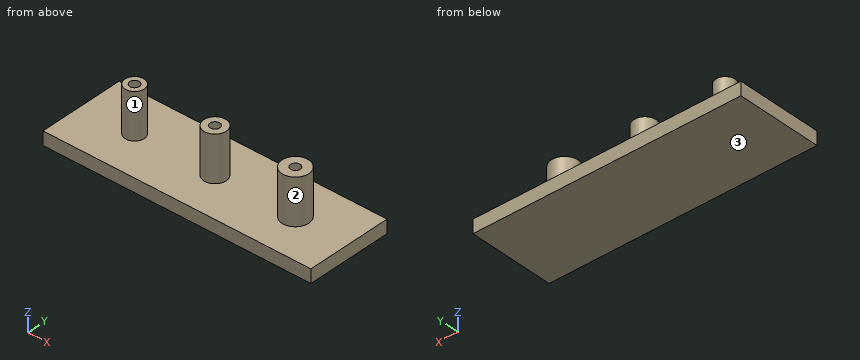
Autodesk Fusion 360 part; units mm, degrees
sketch "Esquisse1" plane through (0, 0, 0) normal (0, 0, 1) x (1, 0, 0)
  line L0 (0, 0) -> (50, 0)
  line L1 (50, 0) -> (50, 16)
  line L2 (50, 16) -> (0, 16)
  line L3 (0, 16) -> (0, 0)
  dimension "d7" = 50
  dimension "d8" = 16
extrude "Extrusion1" add sketch "Esquisse1" along normal blind 2.5
sketch "Esquisse2" plane through (0, 0, 2.5) normal (0, 0, 1) x (-1, 0, 0)
  line L0 (0, -16) -> (0, 0)
  line L1 (0, 0) -> (-50, 0)
  line L2 (-50, 0) -> (-50, -16)
  line L3 (-50, -16) -> (0, -16)
  circle A0 centre (-10, -8) radius 1.8
  dimension "d11" = 3.6
  dimension "d12" = 8
  dimension "d13" = 10
extrude "Extrusion2" add sketch "Esquisse2" along normal blind 8.5 contours A0
sketch "Esquisse3" plane through (0, 0, 2.5) normal (0, 0, 1) x (-1, 0, 0)
  circle A0 centre (-10, -8) radius 1.8
  line L0 (0, -16) -> (0, 0)
  line L1 (0, 0) -> (-50, 0)
  line L2 (-50, 0) -> (-50, -16)
  line L3 (-50, -16) -> (0, -16)
  circle A1 centre (-25, -8) radius 2.1
  dimension "d16" = 4.2
  dimension "d17" = 8
  dimension "d18" = 25
extrude "Extrusion3" add sketch "Esquisse3" along normal blind 8.5 contours A1
sketch "Esquisse4" plane through (0, 0, 2.5) normal (0, 0, 1) x (-1, 0, 0)
  circle A0 centre (-25, -8) radius 2.1
  circle A1 centre (-10, -8) radius 1.8
  line L0 (0, -16) -> (0, 0)
  line L1 (0, 0) -> (-50, 0)
  line L2 (-50, 0) -> (-50, -16)
  line L3 (-50, -16) -> (0, -16)
  circle A2 centre (-40, -8) radius 2.5
  dimension "d21" = 5
  dimension "d22" = 8
  dimension "d23" = 40
extrude "Extrusion4" add sketch "Esquisse4" along normal blind 8.5 contours A2
sketch "Esquisse5" plane through (0, 0, 11) normal (0, 0, 1) x (-1, 0, 0)
  circle A0 centre (-10, -8) radius 1.8
  circle A1 centre (-10, -8) radius 0.9
  dimension "d26" = 1.8
extrude "Extrusion5" cut sketch "Esquisse5" against normal blind 6 contours A1
pattern_linear "Réseau R1" count 3 spacing 15 along (1, 0, 0) of "Extrusion5"
equation "l_plaque = 50 mm"
equation "w_plaque = 16 mm"
equation "ep_plaque = 2.5 mm"
equation "h_plot = 8.5 mm"
equation "d_pilote = 1.8 mm"
equation "p_pilote = 6 mm"
equation "d7 = l_plaque"
equation "d8 = w_plaque"
equation "d9 = ep_plaque"
equation "d14 = h_plot"
equation "d19 = h_plot"
equation "d24 = h_plot"
equation "d26 = d_pilote"
Source: CAD feature listing. Evaluate the final solid. Frame: model axes, mm. Face numbers are marked on the shaded views. Coordinates: 2 decimals unless noted, no trailing zeros. Order: outer loops, then holes, each group sorted by start corner. A loop starts at its lowest first (then second) coordinate and runs counter-clockwise, first axis right, second up. Notation, with made-up numbers: (75, -25.5) - (94, -25.5) arc R26 ccw to (94, -4.5) - close; hole circle Ø1 at (10.25, -22.75). An arc over 180 degrees is marked (long way). One line per item, written item: value.
1) Contact query for flat-ended pins moving along their axis: pin 1 (1.6 mm diameter, centred on x = 40, y = 8, fed in from +Z); pin 2 (3 mm diameter, centred on x = 20.5, y = 10.5, fed in from +Z); pin 3 (2 mm diameter, centred on y = 10.5, z = 9.5, fed in from +X). Output: stop coordinate, or through.
Computed values:
pin 1: stops at z = 5
pin 2: stops at z = 2.5
pin 3: stops at x = 42
2) Cut plane A-A on z = 7. Output: boundary loops of the cut face in (x, y), plus the area to 3 significant figures.
Computed values:
outline: circle Ø3.6 at (10, 8); circle Ø4.2 at (25, 8); circle Ø5 at (40, 8); hole circle Ø1.8 at (10, 8); hole circle Ø1.8 at (25, 8); hole circle Ø1.8 at (40, 8)
area: 36.0 mm^2
3) Ray query, line 1 (X direction, y = 8, z = 6.75); line 2 (Y direction, x = 40, z = 9); line 3 (Y direction, x = 25, z = 9.25). Return the intervals inside material, ascending. Write a range as [from, to].
Computed values:
line 1: x = [8.2, 9.1], [10.9, 11.8], [22.9, 24.1], [25.9, 27.1], [37.5, 39.1], [40.9, 42.5]
line 2: y = [5.5, 7.1], [8.9, 10.5]
line 3: y = [5.9, 7.1], [8.9, 10.1]
4) Cut plane C-C on x = 25. Output: boundary loops of the cut face in (y, z), plus the area to 3 significant figures.
Computed values:
outline: (0, 0) - (16, 0) - (16, 2.5) - (10.1, 2.5) - (10.1, 11) - (8.9, 11) - (8.9, 5) - (7.1, 5) - (7.1, 11) - (5.9, 11) - (5.9, 2.5) - (0, 2.5) - close
area: 64.9 mm^2
5) Cut plane B-B on y = 8. Output: boundary loops of the cut face in (x, z).
Computed values:
outline: (0, 0) - (50, 0) - (50, 2.5) - (42.5, 2.5) - (42.5, 11) - (40.9, 11) - (40.9, 5) - (39.1, 5) - (39.1, 11) - (37.5, 11) - (37.5, 2.5) - (27.1, 2.5) - (27.1, 11) - (25.9, 11) - (25.9, 5) - (24.1, 5) - (24.1, 11) - (22.9, 11) - (22.9, 2.5) - (11.8, 2.5) - (11.8, 11) - (10.9, 11) - (10.9, 5) - (9.1, 5) - (9.1, 11) - (8.2, 11) - (8.2, 2.5) - (0, 2.5) - close
6) Mould query, pull axis X, two halves, no side actions, for the marked faces 1, 2 and 3. Classes: released by +X, released by -X, zero draft, split by the parting line, or undercut.
Computed values:
face 1: undercut
face 2: undercut
face 3: zero draft
7) Cut plane D-D on x = 10. Output: boundary loops of the cut face in (y, z), plus the area to 3 significant figures.
Computed values:
outline: (0, 0) - (16, 0) - (16, 2.5) - (9.8, 2.5) - (9.8, 11) - (8.9, 11) - (8.9, 5) - (7.1, 5) - (7.1, 11) - (6.2, 11) - (6.2, 2.5) - (0, 2.5) - close
area: 59.8 mm^2
